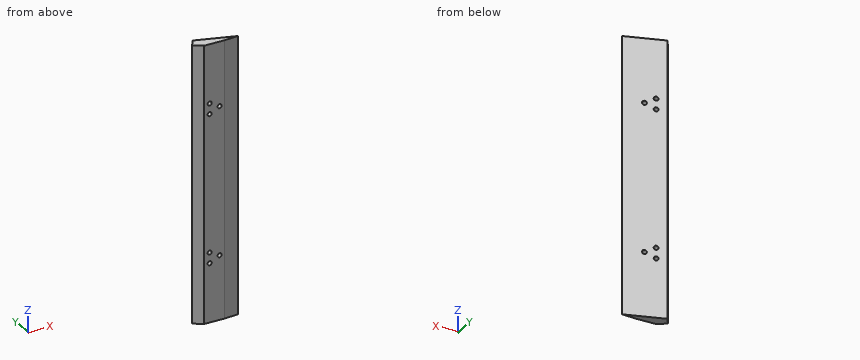
```python
from build123d import *

# Parameters (mm, degrees)
EXTRUDE_1_DEPTH     = 100
SKETCH_2_R          = 1.5
CUT_EXTRUDE_1_DEPTH = 102.998720838


with BuildPart() as part:
    # 草图1 → 凸台-拉伸1 (new, symmetric)
    with BuildSketch(Plane.XY):
        Polygon((-7.5, 0), (7.5, 0), (17.60781312, 0.755729128), (-10.342998863, 9.680081085), (-13.930964167, 4.246815329), align=None)
    extrude(amount=EXTRUDE_1_DEPTH, both=True)

    # 草图2 → 切除-拉伸1 (cut, through all)
    with BuildSketch(Plane.XZ):
        with Locations(Location((3.794045685, 53.578973455, 0), (0, 0, 270))):
            Circle(SKETCH_2_R)
        with Locations(Location((3.794045685, -53.578973455, 0), (0, 0, 270))):
            Circle(SKETCH_2_R)
        with Locations(Location((-3.452778586, 57.415298026, 0), (0, 0, 270))):
            Circle(SKETCH_2_R)
        with Locations(Location((-3.452778586, 49.742648885, 0), (0, 0, 270))):
            Circle(SKETCH_2_R)
        with Locations(Location((-3.452778586, -49.742648885, 0), (0, 0, 270))):
            Circle(SKETCH_2_R)
        with Locations(Location((-3.452778586, -57.415298026, 0), (0, 0, 270))):
            Circle(SKETCH_2_R)
    extrude(amount=-CUT_EXTRUDE_1_DEPTH, mode=Mode.SUBTRACT)


solid = part.part
```
Could you check a few things on this model? Use its own coordinates, in mm. Coordinates: 2 decimals unless noted, no trailing zeros. Write each loop counter-clockwise with the first axis right and the second up, starting at its lowest first coordinate (ties: lowest second). Pieces come first, ordered by that corner, then holes. Notation, with made-up numbers: (-27.75, 84.25) -> (4.25, 84.25) arc R33 cw to (4.25, 120.25) -> close; hole circle Ø1 at (52.25, 43). An arc over 180 degrees is marked (long way). Write item = value, one per line. Start each with the question number.
(1) I want a section at A-A (y = 2.5). Please give me the cut outline in (x, z), plus the area to 3 significant figures.
(2) I want a section at C-C (x = 10). Please give me the cut outline in (y, z).
(3) I need wall thicknesses on line 1 (Z direction, x = 5, y = 1.25); line 2 (Y direction, x = 11.5, z = 8); line 3 (Y direction, x = -11, z = -74). Which ranges of each line are inside material? Lowest first, please. Write a range as [from, to].
(4) Will these pins go through, and if not, where does the flat tip stop? pin 1 (4 mm diameter, centred on x = 3.79, z = 53.58, fed in from +Y); pin 2 (1 mm diameter, centred on x = 5, z = 71, fed in from +Y); pin 3 (2.5 mm diameter, centred on x = -3.45, z = -49.74, fed in from +Y); pin 4 (4 mm diameter, centred on x = -3.45, z = 49.74, fed in from +Y).
(5) I want a section at B-B (z = 4.5). Please give me the cut outline in (x, y), plus the area to 3 significant figures.
Result set:
q1.outline = (-11.29, -100) -> (12.14, -100) -> (12.14, 100) -> (-11.29, 100) -> close; hole circle Ø3 at (-3.45, -57.42); hole circle Ø3 at (-3.45, -49.74); hole circle Ø3 at (-3.45, 49.74); hole circle Ø3 at (-3.45, 57.42); hole circle Ø3 at (3.79, -53.58); hole circle Ø3 at (3.79, 53.58)
q1.area = 4,640 mm2
q2.outline = (0.19, -100) -> (3.18, -100) -> (3.18, 100) -> (0.19, 100) -> close
q3.line_1 = [-100, -54.47], [-52.69, 52.69], [54.47, 100]
q3.line_2 = [0.3, 2.71]
q3.line_3 = [2.31, 8.69]
q4.pin_1 = 5.81
q4.pin_2 = 4.94
q4.pin_3 = through
q4.pin_4 = 8.12
q5.outline = (-13.93, 4.25) -> (-7.5, 0) -> (7.5, 0) -> (17.61, 0.76) -> (-10.34, 9.68) -> close
q5.area = 153 mm2
